Study the drawing (mm; zero at the part's minimum x, y, z) and answer. Round coordinates to 2 decimals unless told otherwise and drop trailing zeros. Write each loop counter-clockwise with the first axis right and the second up, starting at its lowest first coordinate (ties: lowest second). Pieces come first, ordered by that corner, then holes.
(1) A cutting plane is placed at D-D, the plane y = 26.5. Give the vertices of the cut face in (x, z), and give its area (3 significant figures).
(2) Find the intervals of material crossed by probe 1 along Y at (x, z) = (41.5, 37); probe 2 along Y at (x, z) = (50.5, 25.5); probe 3 along X at (y, z) = (49, 25), in increasing order.
(3) A cutting plane is placed at C-C, the plane z = 9. Give the vertices of the cut face in (x, y), and give its area (3 significant figures).
(4) Each of these flat-tipped pins is pushed along its axis until it touches: pin 1 Ø6 at (x, z) = (42, 37) entering from +Y; pin 2 Ø1.5 at (x, y) = (51.5, 3) entering from +Z; pin 3 Ø1.6 at (y, z) = (3, 27.5) entering from +X. Where does it stop, or does it pass through?
(5) A cutting plane is placed at A-A, the plane y = 2.5. Give the vertices of the cut face in (x, z) (1 decimal).
(6) A cutting plane is placed at B-B, the plane x = 25. Give the vertices of the cut face in (y, z), and give its area (4 significant figures).
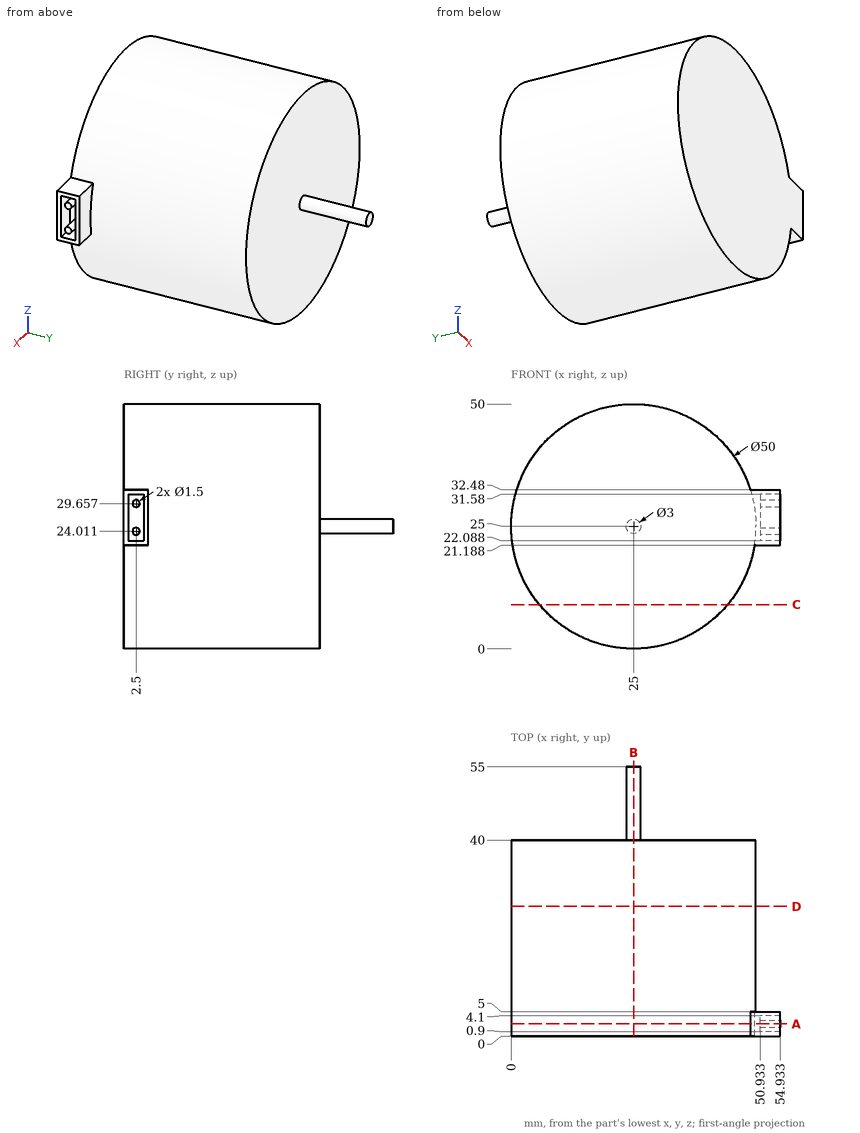
Solutions:
1. outline: circle Ø50 at (25, 25)
1. area: 1,960 mm2
2. probe 1: y = 0 to 40
2. probe 2: y = 0 to 5
2. probe 3: x = 23.5 to 26.5
3. outline: (5.79, 0) - (44.21, 0) - (44.21, 40) - (5.79, 40) - close
3. area: 1,540 mm2
4. pin 1: stops at y = 40
4. pin 2: stops at z = 32.48
4. pin 3: stops at x = 50.93
5. outline: (48.9, 32.5) arc R25 ccw (long way) to (49.7, 21.2) - (54.9, 21.2) - (54.9, 22.1) - (50.9, 22.1) - (50.9, 23.3) - (54.9, 23.3) - (54.9, 24.8) - (50.9, 24.8) - (50.9, 28.9) - (54.9, 28.9) - (54.9, 30.4) - (50.9, 30.4) - (50.9, 31.6) - (54.9, 31.6) - (54.9, 32.5) - close
6. outline: (0, 0) - (40, 0) - (40, 23.5) - (55, 23.5) - (55, 26.5) - (40, 26.5) - (40, 50) - (0, 50) - close
6. area: 2,045 mm2
